```python
from build123d import *

# Parameters (mm, degrees)
CROQUIS1_W              = 45
CROQUIS1_H              = 30
SALIENTE_EXTRUIR1_DEPTH = 9
CROQUIS2_R              = 2.5
CROQUIS2_W              = 15
CROQUIS2_H              = 15
CORTAR_EXTRUIR1_DEPTH   = 10


with BuildPart() as part:
    # Croquis1 → Saliente-Extruir1 (new body)
    with BuildSketch(Plane(origin=(0, 0, 0), x_dir=(1, 0, 0), z_dir=(0, 1, 0))):
        with Locations((22.5, 15)):
            Rectangle(CROQUIS1_W, CROQUIS1_H)
    extrude(amount=SALIENTE_EXTRUIR1_DEPTH)

    # Croquis2 → Cortar-Extruir1 (cut)
    with BuildSketch(Plane(origin=(0, 9, 0), x_dir=(1, 0, 0), z_dir=(0, 1, 0))):
        with Locations(Location((5, 22, 0), (0, 0, 270))):
            Circle(CROQUIS2_R)
        with Locations(Location((5, 8, 0), (0, 0, 270))):
            Circle(CROQUIS2_R)
        with Locations(Location((40, 8, 0), (0, 0, 90))):
            Circle(CROQUIS2_R)
        with Locations(Location((40, 22, 0), (0, 0, 90))):
            Circle(CROQUIS2_R)
        with Locations((22.5, 15)):
            Rectangle(CROQUIS2_W, CROQUIS2_H)
    extrude(amount=-CORTAR_EXTRUIR1_DEPTH, mode=Mode.SUBTRACT)


solid = part.part
```
Design review of the part built by this model. Coordinates are the model's own, in mm. A direction names the side the tool comes from. Coordinates: 2 decimals unless noted, no trailing zeros. Order: outer loops, then holes, each group sorted by start corner. A loop starts at its lowest first (then second) coordinate and runs counter-clockwise, first axis right, second up. Notation, with made-up numbers: (33, -8) -> (50, -8) arc R19 cw to (50, 1) -> close; hole circle Ø5 at (26.25, 45.5). An arc over 180 degrees is marked (long way). One line per item, written item: value. Start each with the question number.
Q1. Take a section at D-D, the plane z = -22. State the section outline as (x, y) points.
Q2. Mouldability with a two-part tool opening along X and no side actions: class faces 1 (the flat face through (22, 4, -30)), 2 (the flat face through (0, 4, -15)), 3 (the flat face through (22, 5, -7.5)) as pulls with the +X half, pulls with the -X half, needs draft (parallel to the pull), parting line crosses it, or undercut.
Q3. For probe 1 along Z at (x, y) = (40, 4.5); probe 2 along X at (y, z) = (3, -22); probe 3 along Z at (x, y) = (29, 6), list the stretches that pass through material, from the lowest coordinate up.
Q4. Take a section at A-A, the plane z = -14. State the section outline as (x, y) points, then the cut area to 3 significant figures.
Q5. Take a section at B-B, the plane y = 6.5. State the section outline as (x, z) points, then the cut area to 3 significant figures.
Q6. Insertion check: pin 1 Ø5 at (x, y) = (23.5, 2) entering from +Z; pin 2 Ø3 at (x, z) = (40, -8) entering from -Y. Each pin has a flat end and moves straight along its axis. Give the tip position at first contact, or say it passes through.
Q7. Tool access review of faces 4 (the flat face through (15, 5, -15)), 5 (the flat face through (22, 4, 0)): name each direction out of +Z, -Z, +X, -X, +Y, -Y from which nothing blocks a thin tool from reaching the whole face with its end or side.
Q8. Take a section at C-C, the plane x = 40. State the section outline as (y, z) points, then the cut area to 3 significant figures.
Values follow:
1. outline: (0, 0) -> (2.5, 0) -> (2.5, 9) -> (0, 9) -> close; (7.5, 0) -> (15, 0) -> (15, 9) -> (7.5, 9) -> close; (30, 0) -> (37.5, 0) -> (37.5, 9) -> (30, 9) -> close; (42.5, 0) -> (45, 0) -> (45, 9) -> (42.5, 9) -> close
2. face 1: needs draft
2. face 2: pulls with the -X half
2. face 3: undercut
3. probe 1: z = -30 to -24.5, -19.5 to -10.5, -5.5 to 0
3. probe 2: x = 0 to 2.5, 7.5 to 15, 30 to 37.5, 42.5 to 45
3. probe 3: z = -30 to -22.5, -7.5 to 0
4. outline: (0, 0) -> (15, 0) -> (15, 9) -> (0, 9) -> close; (30, 0) -> (45, 0) -> (45, 9) -> (30, 9) -> close
4. area: 270 mm2
5. outline: (0, -30) -> (45, -30) -> (45, 0) -> (0, 0) -> close; hole circle Ø5 at (5, -22); hole circle Ø5 at (5, -8); hole (15, -22.5) -> (30, -22.5) -> (30, -7.5) -> (15, -7.5) -> close; hole circle Ø5 at (40, -22); hole circle Ø5 at (40, -8)
5. area: 1,050 mm2
6. pin 1: stops at z = 0
6. pin 2: passes through
7. face 4: +Y, -Y
7. face 5: +Z, +X, -X, +Y, -Y
8. outline: (0, -30) -> (9, -30) -> (9, -24.5) -> (0, -24.5) -> close; (0, -19.5) -> (9, -19.5) -> (9, -10.5) -> (0, -10.5) -> close; (0, -5.5) -> (9, -5.5) -> (9, 0) -> (0, 0) -> close
8. area: 180 mm2
